For this review, use the dimensioned drawing (mm, ordinates from the lowest corner) and the shaded views. A direction names the side the tool comes from. Round coordinates to 2 decimals unless told otherwise and drop trailing zeros. Loops run counter-clockwise (first coordinate to the right, second up) from the corner with the lowest first, then second, coordinate; pieces in that order, holes last.
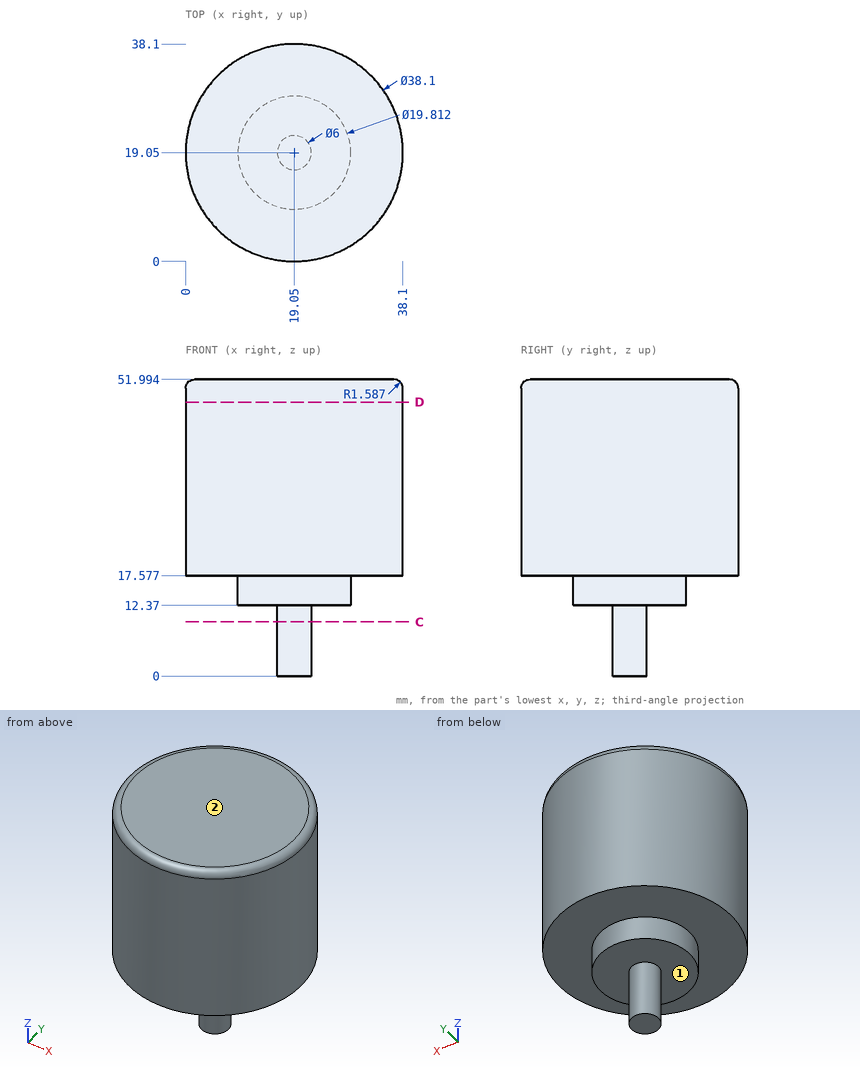
(1) For L1, parallel to Z at x = 31, y = 20; L2, parallel to Z at x = 26.5, y = 18.5; L3, parallel to X at y = 19.5, z = 48.5 (1 decimal), list the stretches that pass through material, from the lowest coordinate up.
(2) Add section D-D (z = 48). Give the boundary of the cut face in (x, y).
(3) For the marked faces 1 and 2, list the 3-axis set-ups (+Z, -Z, +X, -X, +Y, -Y) from which the entire face can be reached by the end or side of a thin tool; tool diameter is ignored.
(4) Insertion check: pin 1 Ø2 at (x, z) = (15.5, 38.5) entering from +Y; pin 2 Ø3 at (y, z) = (33, 22) entering from +X; pin 3 Ø6 at (x, y) = (28, 8) entering from -Z. Each pin has a flat end and moves straight along its axis. Give the tip position at first contact, or say it passes through.
(5) Add section C-C (z = 9.5). Give the boundary of the cut face in (x, y).
Outcome:
1. L1: z = 17.58 to 51.99
1. L2: z = 12.37 to 51.99
1. L3: x = 0 to 38.1
2. outline: circle Ø38.1 at (19.05, 19.05)
3. face 1: -Z
3. face 2: +Z, +X, -X, +Y, -Y
4. pin 1: stops at y = 37.93
4. pin 2: stops at x = 33.47
4. pin 3: stops at z = 17.58
5. outline: circle Ø6 at (19.05, 19.05)
